For this review, take the finished solid that the model builds, in its own axes (mm). A direction names the side the tool comes from. Round coordinates to 2 decimals unless told otherwise and drop trailing zeros. Loops run counter-clockwise (first coordinate to the right, second up) from the corner with the lowest first, then second, coordinate; pieces in that order, holes last.
Autodesk Inventor part; units mm, degrees
ref_plane "Work Plane2" through (-11, -11, -12.1) normal (0, 0, 1) x (1, 0, 0)
ref_plane "Work Plane3" through (-21, -21, -14.1) normal (0, 0, 1) x (1, 0, 0)
ref_plane "Work Plane5" through (-21, -21, -14.1) normal (0, 0, 1) x (1, 0, 0)
ref_plane "Work Plane1" through (0, 0, 0.1) normal (0, 0, 1) x (1, 0, 0)
sketch "Sketch2" plane through (0, 0, 0.1) normal (0, 0, 1) x (1, 0, 0)
  arc A0 (-1.5411, 2.125) -> (1.5411, 2.125) centre (0, 0) ccw construction
  line L0 (-1.5411, 2.125) -> (1.5411, 2.125) construction
  circle A1 centre (0, 0) radius 8 construction
  line L1 (1.5, 2) -> (-1.5, 2) construction
  arc A2 (-1.5, 2) -> (1.5, 2) centre (0, 0) ccw construction
  circle A3 centre (0, 0) radius 11
  circle A4 centre (-15.5, -15.5) radius 1.75 construction
  circle A5 centre (15.5, -15.5) radius 1.75 construction
  circle A6 centre (15.5, 15.5) radius 1.75 construction
  circle A7 centre (-15.5, 15.5) radius 1.75 construction
  line L2 (-21, 21) -> (21, 21) construction
  line L3 (-21, -21) -> (-21, 21) construction
  line L4 (21, -21) -> (-21, -21) construction
  line L5 (21, 21) -> (21, -21) construction
  line L6 (-11, 0) -> (-11, 21)
  line L7 (-11, 21) -> (11, 21)
  line L8 (11, 21) -> (11, 0)
  circle A8 centre (0, 0) radius 2.625
  dimension "d0" = 5.25
extrude "Extrusion1" add sketch "Sketch2" along normal blind 5
sketch "Sketch3" plane through (0, 0, 0.1) normal (0, 0, -1) x (-1, 0, 0)
  circle A0 centre (0, 13.698) radius 2.2
  circle A1 centre (0, 13.698) radius 2
  point P0 (0, 0)
  dimension "d3" = 4
extrude "Extrusion2" cut sketch "Sketch3" against normal blind 3 contours A1
sketch "Sketch4" plane through (0, 13.698, 3.1) normal (0, 0, -1) x (-1, 0, 0)
  circle A0 centre (0, 0) radius 1
  circle A1 centre (0, 0) radius 2
  point P0 (0, -13.698)
  dimension "d6" = 2
extrude "Extrusion3" cut sketch "Sketch4" against normal through all contours A0
sketch "Sketch5" plane through (0, 0, 0.1) normal (0, 0, -1) x (-1, 0, 0)
  circle A0 centre (0, 0) radius 8 construction
  line L0 (-8, 0) -> (-8, 21) construction
  line L1 (-11, 21) -> (11, 21) construction
  line L2 (8, 0) -> (8, 21) construction
  line L3 (-8.5, 0) -> (-8.5, 21) construction
  line L4 (8.5, 0) -> (8.5, 21) construction
  circle A1 centre (0, 0) radius 8.5 construction
  line L5 (-8.5, 0) -> (-12, 0)
  line L6 (-12, 0) -> (-12, 21)
  line L7 (-12, 21) -> (-8.5, 21)
  line L8 (-8.5, 21) -> (-8.5, 0)
  line L9 (8.5, 0) -> (12, 0)
  line L10 (12, 0) -> (12, 21)
  line L11 (12, 21) -> (8.5, 21)
  line L12 (8.5, 21) -> (8.5, 0)
  line L13 (11, 21) -> (-11, 21)
  dimension "d9" = 0.5
  dimension "d10" = 0.5
  dimension "d11" = 0.5
  dimension "d12" = 3.5
  dimension "d13" = 3.5
ref_plane "Work Plane2" through (-11, -11, -12.1) normal (0, 0, 1) x (1, 0, 0)
extrude "Extrusion4" add sketch "Sketch5" along normal up to surface (12.2 mm away)
sketch "Sketch6" plane through (0, 0, 0.1) normal (0, 0, 1) x (1, 0, 0)
  line L0 (-11, 0) -> (-11, 21)
  line L1 (-11, 21) -> (-12, 21)
  line L2 (-12, 21) -> (-12, 0)
  line L3 (-12, 0) -> (-11, 0)
  line L4 (11, 21) -> (11, 0)
  line L5 (11, 0) -> (12, 0)
  line L6 (12, 0) -> (12, 21)
  line L7 (12, 21) -> (11, 21)
  point P0 (0, 0)
extrude "Extrusion5" add sketch "Sketch6" along normal up to surface (5 mm away)
fillet "Fillet1" radius 2 2 edges at (11, 0, 2.6) (-11, 0, 2.6)
sketch "Sketch7" plane through (12, 0, -12.1) normal (0, 0, -1) x (-1, 0, 0)
  circle A0 centre (12, 0) radius 11
  line L0 (33, 21) -> (-9, 21) construction
  circle A1 centre (27.5, -15.5) radius 1.75 construction
  circle A2 centre (-3.5, -15.5) radius 1.75 construction
  circle A3 centre (-3.5, 15.5) radius 1.75 construction
  circle A4 centre (27.5, 15.5) radius 1.75 construction
  line L1 (33, 21) -> (-9, 21) construction
  line L2 (-9, 21) -> (-9, -21) construction
  line L3 (-9, -21) -> (33, -21) construction
  line L4 (33, -21) -> (33, 21) construction
  circle A5 centre (-3.5, 15.5) radius 1.75
  arc A6 (-3.5, 21) -> (-3.5, 10) centre (-3.5, 15.5) ccw
  line L5 (0, 21) -> (0, 0)
  arc A7 (0, 6.5) -> (-3.5, 10) centre (-3.5, 6.5) ccw
  line L6 (24, 21) -> (0, 21)
  line L7 (-3.5, 21) -> (0, 21)
  arc A8 (1.1058, -1.5218) -> (0, 0) centre (-0.875, -1.7984) ccw
  arc A9 (24, 0) -> (22.8942, -1.5218) centre (24.875, -1.7984) ccw
  line L8 (24, 0) -> (24, 21)
  circle A10 centre (12, 0) radius 12
  line L9 (0, 0) -> (3.5, 0)
  line L10 (0, 6.5) -> (0, 0)
  line L11 (0, 21) -> (12, 21)
  line L12 (20.5, 21) -> (3.5, 21)
  line L13 (12, 21) -> (12, 14.698)
  circle A11 centre (12, 13.698) radius 1
  line L14 (12, 12.698) -> (12, 12)
  arc A12 (12, 12) -> (0, 0) centre (12, 0) ccw
  arc A13 (12, 14.698) -> (12, 12.698) centre (12, 13.698) ccw
  point P0 (12, 0)
  point P1 (-3.125, 21)
ref_plane "Work Plane3" through (-21, -21, -14.1) normal (0, 0, 1) x (1, 0, 0)
extrude "Extrusion6" add sketch "Sketch7" along normal up to surface (2 mm away) contours L5 L6 L13 A11 L14 A10 | A7 A6 L7 L5
mirror "Mirror1" about plane through (0, 14.698, -12.1) normal (-1, 0, 0) of "Extrusion6"
ref_plane "Work Plane4" through (0, 13.698, -11.1) normal (0, 0, -1) x (-1, 0, 0)
sketch "Sketch9" plane through (0, 13.698, -11.1) normal (0, 0, -1) x (-1, 0, 0)
  circle A0 centre (0, 0) radius 5.2
  circle A1 centre (0, 0) radius 2
  line L0 (-8.5, 7.302) -> (8.5, 7.302)
  line L1 (8.5, 7.302) -> (8.5, -5.2275)
  arc A2 (8.5, -5.2275) -> (-8.5, -5.2275) centre (0, -13.698) ccw
  line L2 (-8.5, -5.2275) -> (-8.5, 7.302)
  circle A3 centre (0, 0) radius 1
  arc A4 (8.5, -5.2275) -> (-8.5, -5.2275) centre (0, -13.698) ccw
  arc A5 (8.5, -5.2275) -> (0.9883, -1.7388) centre (0, -13.698) ccw
  arc A6 (-0.9883, -1.7388) -> (-8.5, -5.2275) centre (0, -13.698) ccw
  arc A7 (0.9883, -1.7388) -> (-0.9883, -1.7388) centre (0, 0) ccw
  line L3 (-12, 7.302) -> (-12, -7.198)
  arc A8 (-12, -7.198) -> (-15.5, -3.698) centre (-15.5, -7.198) ccw
  arc A9 (-15.5, 7.302) -> (-15.5, -3.698) centre (-15.5, 1.802) ccw
  line L4 (-12, 7.302) -> (-15.5, 7.302)
  point P0 (0, -13.698)
  dimension "d26" = 4
extrude "Extrusion8" add sketch "Sketch9" along normal up to surface (1 mm away) contours A0 A2 A1 | A0 A2 L2 L0 L1 | A1 A2 | A3 picked at (-3.5209, -0.8252) picked at (-0.5576, -1.4588)
sketch "Sketch10" plane through (12, 0, -12.1) normal (0, 0, 1) x (1, 0, 0)
  circle A0 centre (-12, 13.698) radius 1
  circle A1 centre (-12, 13.698) radius 2
  point P0 (-12, 0)
  dimension "d29" = 4
extrude "Extrusion9" cut sketch "Sketch10" against normal through all
sketch "Sketch11" plane through (-8.5, 0, -12.1) normal (0, 0, -1) x (-1, 0, 0)
  circle A0 centre (-8.5, 0) radius 11 construction
  arc A1 (-20.5, 0) -> (-20.5, 0) centre (-8.5, 0) ccw construction
  arc A2 (3.5, 0) -> (-20.5, 0) centre (-8.5, 0) ccw construction
  arc A3 (-9.4883, 11.9592) -> (-17, 8.4705) centre (-8.5, 0) ccw construction
  arc A4 (-11.5525, 11.6053) -> (-5.4475, 11.6053) centre (-8.5, 19) ccw
  circle A5 centre (-8.5, 13.698) radius 2 construction
  arc A6 (-9.4883, 11.9592) -> (-7.5117, 11.9592) centre (-8.5, 13.698) ccw
  arc A7 (-5.4475, 11.6053) -> (-7.5117, 11.9592) centre (-8.5, 0) ccw
  arc A8 (-9.4883, 11.9592) -> (-11.5525, 11.6053) centre (-8.5, 0) ccw
  point P0 (-8.5, 0)
  dimension "d32" = 8
ref_plane "Work Plane5" through (-21, -21, -14.1) normal (0, 0, 1) x (1, 0, 0)
extrude "Extrusion10" add sketch "Sketch11" along normal up to surface (2 mm away)
sketch "Sketch12" plane through (-8.5, 0, -12.1) normal (0, 0, 1) x (1, 0, 0)
  arc A0 (7.5117, 11.9592) -> (9.4883, 11.9592) centre (8.5, 13.698) ccw
  arc A1 (7.5117, 11.9592) -> (5.4475, 11.6053) centre (8.5, 0) ccw
  arc A2 (5.4475, 11.6053) -> (11.5525, 11.6053) centre (8.5, 19) ccw
  arc A3 (11.5525, 11.6053) -> (9.4883, 11.9592) centre (8.5, 0) ccw
  point P0 (8.5, 0)
extrude "Extrusion11" add sketch "Sketch12" along normal up to surface (1 mm away)
sketch "Sketch13" plane through (12, 0, -12.1) normal (0, 0, 1) x (1, 0, 0)
  line L0 (0, 21) -> (0, 6.5)
  arc A0 (3.5, 10) -> (0, 6.5) centre (3.5, 6.5) ccw
  arc A1 (3.5, 10) -> (3.5, 21) centre (3.5, 15.5) ccw
  line L1 (0, 21) -> (3.5, 21)
  circle A2 centre (3.5, 15.5) radius 1.75
  line L2 (-24, 6.5) -> (-24, 21)
  line L3 (-24, 21) -> (-27.5, 21)
  arc A3 (-27.5, 21) -> (-27.5, 10) centre (-27.5, 15.5) ccw
  arc A4 (-24, 6.5) -> (-27.5, 10) centre (-27.5, 6.5) ccw
  circle A5 centre (-27.5, 15.5) radius 1.75
  point P0 (-12, 0)
extrude "Extrusion12" add sketch "Sketch13" along normal blind 2
properties part number "Bracket"
(1) Add section A-A (z = -6). Give the boundary of the cut face in (x, y), plus the area to 3 significant figures.
(2) Add section C-C (y = 2). Give the boundary of the cut face in (x, z), plus the area to 3 significant figures.
(3) For faces 4 (the cylindrical face through (-9.44, 7.41, -13.09)), 5 (the cylindrical face through (-1.908, 14.299, 1.579)), 6 (the flat face through (0, 14, -12.1)), 7 (the flat face through (17.44, 15.46, -10.1)), list the 3-axis set-ups (+Z, -Z, +X, -X, +Y, -Y) from which the entire face can be reached by the end or side of a thin tool; tool diameter is ignored.
(4) Add section D-D (x = 0). Give the boundary of the cut face in (y, z) (3 decimals).
(5) Insertion check: pin 1 Ø2 at (y, z) = (8, -6) entering from +X; pin 2 Ø5 at (y, z) = (5.5, 3) entering from -X; pin 3 Ø1 at (x, y) = (10.5, 3.5) entering from -Z. Each pin has a flat end and moves straight along its axis. Give the tip position at first contact, or say it passes through.
(6) Add section B-B (x = 15). Give the boundary of the cut face in (y, z), plus the area to 3 significant figures.
(7) For L1, parallel to Y at x = 0, z = 1.7 (3 decimals); L2, parallel to Y at x = 0, z = 4.6 (3 decimals); L3, parallel to Y at x = -15.5, z = -12.85, list the stretches that pass through material, from the lowest coordinate up.
(8) The part is to be moulded in two halves that separate along X. For faces 1 (the flat face through (8.5, 11, -6)), 2 (the cylindrical face through (11.25, -0.63, 2.56)), 3 (the flat face through (10, 0, -6)), say which applies: pulls with the +X half, pulls with the -X half, needs draft (parallel to the pull), parting line crosses it, or undercut.
Outcome:
1. outline: (-12, 0) - (-8.5, 0) - (-8.5, 21) - (-12, 21) - close; (8.5, 0) - (12, 0) - (12, 21) - (8.5, 21) - close
1. area: 147 mm2
2. outline: (-12, -14.1) - (-11.83, -14.1) - (-11.83, -12.1) - (-8.5, -12.1) - (-8.5, 0.1) - (-1.7, 0.1) - (-1.7, 5.1) - (-12, 5.1) - close; (1.7, 0.1) - (8.5, 0.1) - (8.5, -12.1) - (11.83, -12.1) - (11.83, -14.1) - (12, -14.1) - (12, 5.1) - (1.7, 5.1) - close
2. area: 189 mm2
3. face 4: -Z, -Y
3. face 5: none
3. face 6: -Z
3. face 7: +Z, +X, +Y, -Y
4. outline: (-11, 0.1) - (-2.625, 0.1) - (-2.625, 5.1) - (-11, 5.1) - close; (2.625, 0.1) - (11.698, 0.1) - (11.698, 3.1) - (12.698, 3.1) - (12.698, 5.1) - (2.625, 5.1) - close; (11, -14.1) - (11.698, -14.1) - (11.698, -11.1) - (11, -11.1) - close; (12, -12.1) - (15.698, -12.1) - (15.698, -14.1) - (21, -14.1) - (21, -11.1) - (12, -11.1) - close; (14.698, 3.1) - (15.698, 3.1) - (15.698, 0.1) - (21, 0.1) - (21, 5.1) - (14.698, 5.1) - close
5. pin 1: stops at x = 12
5. pin 2: stops at x = -12
5. pin 3: stops at z = -12.1
6. outline: (9.96, -14.1) - (13.82, -14.1) - (13.82, -10.1) - (9.96, -10.1) - close; (17.18, -14.1) - (21, -14.1) - (21, -10.1) - (17.18, -10.1) - close
6. area: 30.7 mm2
7. L1: y = -11 to -2.625, 2.625 to 11.698, 15.698 to 21
7. L2: y = -11 to -2.625, 2.625 to 12.698, 14.698 to 21
7. L3: y = 10 to 13.75, 17.25 to 21
8. face 1: undercut
8. face 2: pulls with the +X half
8. face 3: needs draft
